```python
from build123d import *

# Parameters (mm, degrees)
SKETCH1_W           = 30
SKETCH1_H           = 15
SKETCH1_W_2         = 26
SKETCH1_H_2         = 11
BOSS_EXTRUDE1_DEPTH = 10
SKETCH3_R           = 2.5
CUT_EXTRUDE1_DEPTH  = 100
SKETCH5_W           = 300
SKETCH5_H           = 10
BOSS_EXTRUDE2_DEPTH = 10
SKETCH6_W           = 8
SKETCH6_H           = 6
CUT_EXTRUDE2_DEPTH  = 300
SKETCH7_R           = 1.5
SKETCH7_R_2         = 2.5
CUT_EXTRUDE3_DEPTH  = 300
FILLET1_R           = 1.5
SKETCH8_W           = 15
SKETCH8_H           = 6
CUT_EXTRUDE4_DEPTH  = 0.5
SKETCH11_W          = 15
SKETCH11_H          = 6
CUT_EXTRUDE8_DEPTH  = 1
SKETCH9_W           = 15
SKETCH9_H           = 6
CUT_EXTRUDE5_DEPTH  = 0.5


with BuildPart() as part:
    # Sketch1 → Boss-Extrude1 (new body)
    with BuildSketch(Plane.XY):
        with Locations((15, 7.5)):
            Rectangle(SKETCH1_W, SKETCH1_H)
        with Locations((15, 7.5)):
            Rectangle(SKETCH1_W_2, SKETCH1_H_2, mode=Mode.SUBTRACT)
    extrude(amount=BOSS_EXTRUDE1_DEPTH)

    # Sketch3 → Cut-Extrude1 (cut)
    with BuildSketch(Plane(origin=(0, 15, 0), x_dir=(1, 0, 0), z_dir=(0, 1, 0))):
        with Locations(Location((12.5, -5, 0), (0, 0, 270))):
            Circle(SKETCH3_R)
    extrude(amount=-CUT_EXTRUDE1_DEPTH, mode=Mode.SUBTRACT)

    # Sketch5 → Boss-Extrude2 (add)
    with BuildSketch(Plane(origin=(0, 0, 0), x_dir=(-1, 0, 0), z_dir=(0, 0, -1))):
        with Locations((-180, 7.5)):
            Rectangle(SKETCH5_W, SKETCH5_H)
    extrude(amount=-BOSS_EXTRUDE2_DEPTH)

    # Sketch6 → Cut-Extrude2 (cut)
    with BuildSketch(Plane(origin=(330, 0, 0), x_dir=(0, 0, -1), z_dir=(1, 0, 0))):
        with Locations((-6, 7.5)):
            Rectangle(SKETCH6_W, SKETCH6_H)
    extrude(amount=-CUT_EXTRUDE2_DEPTH, mode=Mode.SUBTRACT)

    # Sketch7 → Cut-Extrude3 (cut)
    with BuildSketch(Plane(origin=(0, 2.5, 0), x_dir=(-1, 0, 0), z_dir=(0, -1, 0))):
        with Locations(Location((-272.5, -5, 0), (0, 0, 90))):
            Circle(SKETCH7_R)
        with Locations(Location((-297.5, -5, 0), (0, 0, 90))):
            Circle(SKETCH7_R_2)
        with Locations(Location((-322.5, -5, 0), (0, 0, 90))):
            Circle(SKETCH7_R)
    extrude(amount=-CUT_EXTRUDE3_DEPTH, mode=Mode.SUBTRACT)

    # Fillet1
    fillet1_edges = [part.edges().sort_by_distance(p)[0] for p in [
        (330, 11.5, 10),
        (330, 3.5, 10),
    ]]
    fillet(fillet1_edges, radius=FILLET1_R)

    # Sketch8 → Cut-Extrude4 (cut)
    with BuildSketch(Plane.XY.offset(2)):
        with Locations((49.047215434, 7.5)):
            Rectangle(SKETCH8_W, SKETCH8_H)
    extrude(amount=-CUT_EXTRUDE4_DEPTH, mode=Mode.SUBTRACT)

    # Sketch11 → Cut-Extrude8 (cut)
    with BuildSketch(Plane.XY.offset(2)):
        with Locations((254.956595829, 7.5)):
            Rectangle(SKETCH11_W, SKETCH11_H)
    extrude(amount=-CUT_EXTRUDE8_DEPTH, mode=Mode.SUBTRACT)

    # Sketch9 → Cut-Extrude5 (cut)
    with BuildSketch(Plane.XY.offset(2)):
        with Locations((308.27436269, 7.5)):
            Rectangle(SKETCH9_W, SKETCH9_H)
    extrude(amount=-CUT_EXTRUDE5_DEPTH, mode=Mode.SUBTRACT)


solid = part.part
```
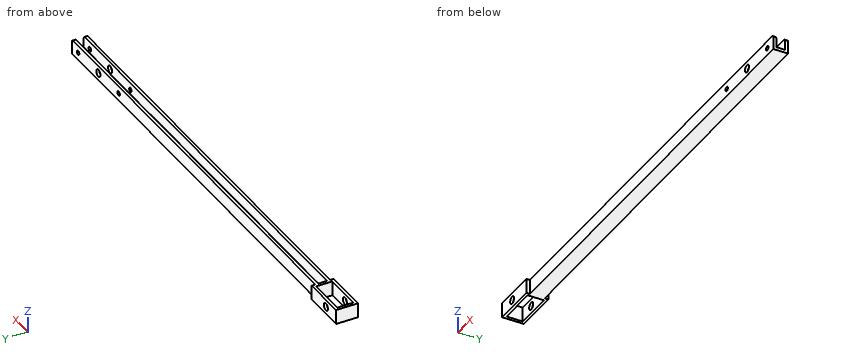
For this review, take the finished solid that the model builds, in its own axes (mm). Round coordinates to 2 decimals unless told otherwise and drop trailing zeros. Write each loop counter-clockwise with the first axis right and the second up, starting at its lowest first coordinate (ties: lowest second). Pieces come first, ordered by that corner, then holes.
1) Insertion check: pin 1 Ø4 at (x, z) = (282, 4.5) entering from -Y; pin 2 Ø5 at (x, z) = (157, 3.5) entering from +Y; pin 3 Ø1.2 at (y, z) = (1.5, 3.5) entering from +X. Each pin has a flat end and moves straight along its axis. Give the tip position at first contact, or say it passes through.
Answer below:
pin 1: stops at y = 2.5
pin 2: stops at y = 12.5
pin 3: stops at x = 30
2) For line 1 along X through (y, z) = (3.2, 5); line 2 along X through (y, z) = (6.5, 6.75); line 3 along Y through (x, z) = (277.5, 6), list the stretches that pass through material, from the lowest coordinate up.
Answer below:
line 1: x = 0 to 2, 28 to 271, 274 to 295, 300 to 321, 324 to 330
line 2: x = 0 to 2, 28 to 30
line 3: y = 2.5 to 4.5, 10.5 to 12.5
3) Take a section at C-C on z = 5. State how many separate pieces and enclosed holes the cut face has, then the cut area to 3 significant figures.
Answer below:
separate pieces: 8
enclosed holes: 0
area: 1,300 mm2
4) Take a section at A-A on y = 7.25. Give the boundary of the cut face in (x, z).
Answer below:
outline: (0, 0) - (2, 0) - (2, 10) - (0, 10) - close; (28, 0) - (330, 0) - (330, 2) - (315.77, 2) - (315.77, 1.5) - (300.77, 1.5) - (300.77, 2) - (262.46, 2) - (262.46, 1) - (247.46, 1) - (247.46, 2) - (56.55, 2) - (56.55, 1.5) - (41.55, 1.5) - (41.55, 2) - (30, 2) - (30, 10) - (28, 10) - close
5) Take a section at B-B on x = 151. Give the boundary of the cut face in (y, z).
Answer below:
outline: (2.5, 0) - (12.5, 0) - (12.5, 10) - (10.5, 10) - (10.5, 2) - (4.5, 2) - (4.5, 10) - (2.5, 10) - close
